Part print with two shaded views. Sizes in mm from the minimum x, y, z corner. A direction names the side the tool comes from. Give positions to 0.01 mm unless a question says otherwise; leave off trailing zeros. Order: outer loops, then holes, each group sorted by start corner. A loop starts at its lowest first (then second) coordinate and runs counter-clockwise, first axis right, second up. Notation, with made-up numbers: (-19.75, 84.25) -> (3.25, 84.25) arc R13 cw to (3.25, 108.25) -> close; hole circle Ø4 at (-10.75, 46). An arc over 180 degrees is marked (long way). Write item = value, one per line. Start each with the question number.
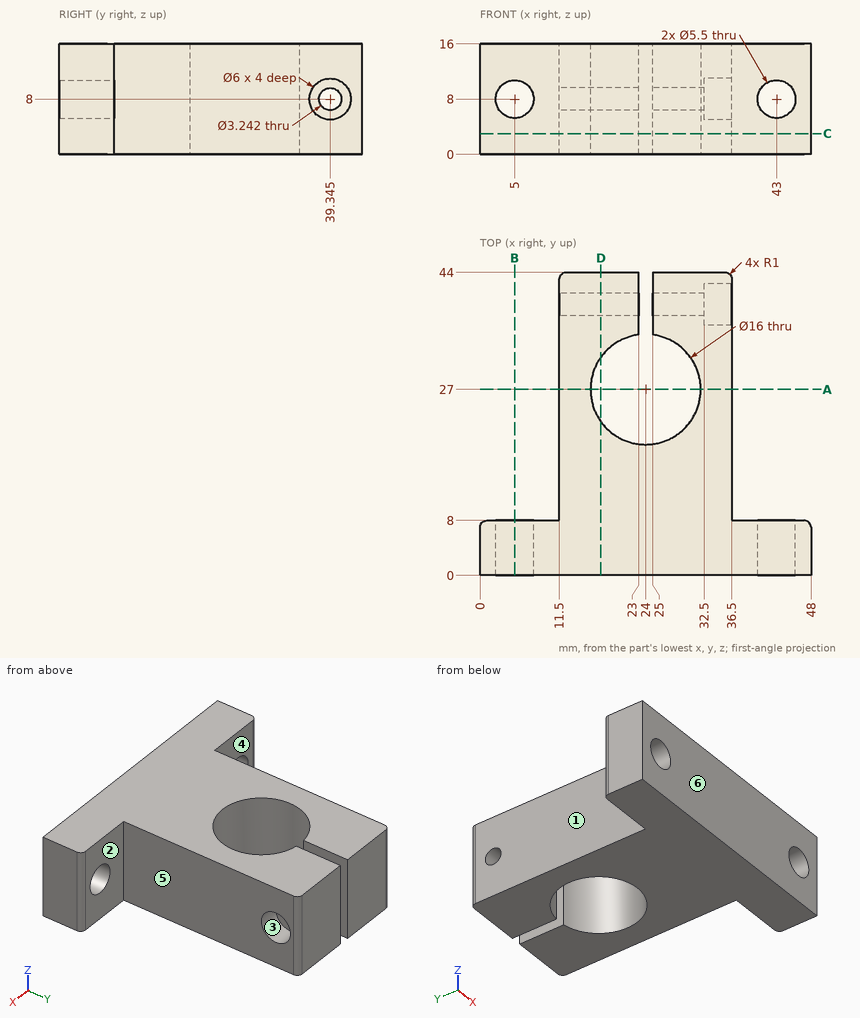
(1) Cut at C-C, the plane z = 3. Give the cut face in (x, y).
(2) Wall check: line 1 (X direction, y = 6, z = 8); line 2 (Y direction, x = 35.1, z = 8) (1 decimal); line 3 (Y direction, x = 25.5, z = 7.75). Give the ranges that are in metal, low to high. Write a range as [from, to].
(3) Mould opens along Y. For the marked faces 1, 2 and 3 say: released by +Y, released by -Y, zero draft, split by the parting line, or undercut.
(4) 3-axis set-ups, long thin cutter, end or side, ignore diameter. For the marked faces 4, 5 and 6: which of +Z, -Z, +X, -X, +Y, -Y reach the whole face in a straight line?
(5) Cut at B-B, the plane x = 5. Give the cut face in (y, z), plus the area to 3 significant figures.
(6) Cut at D-D, the plane x = 17.5. Give the cut face in (y, z) (1 decimal).
(7) Cut at A-A, the plane y = 27. Give the cut face in (x, z).
(8) Flat gauge pins, fed straight in: P1, Ø1.8, axis at y = 40, z = 8.5, coming from the +X side; P2, Ø5.5, axis at y = 39.35, z = 8, coming from the -X side; P3, Ø6.5, axis at x = 43, z = 8, coming from the +Y side; P4, Ø6, axis at y = 6.5, z = 7, coming from the -X side. Where does each tip first touch, or does it go through?
Results:
q1.outline = (0, 0) -> (48, 0) -> (48, 7) arc R1 ccw to (47, 8) -> (36.5, 8) -> (36.5, 43) arc R1 ccw to (35.5, 44) -> (25, 44) -> (25, 34.94) arc R8 cw (long way) to (23, 34.94) -> (23, 44) -> (12.5, 44) arc R1 ccw to (11.5, 43) -> (11.5, 8) -> (1, 8) arc R1 ccw to (0, 7) -> close
q2.line_1 = [0, 2.25], [7.75, 40.25], [45.75, 48]
q2.line_2 = [0, 36.3], [42.3, 44]
q2.line_3 = [0, 19.14], [34.86, 37.74], [40.95, 44]
q3.face_1 = zero draft
q3.face_2 = released by +Y
q3.face_3 = undercut
q4.face_4 = +Z, -Z, -X, +Y
q4.face_5 = +Z, -Z, +X, +Y
q4.face_6 = +Z, -Z, +X, -X, -Y
q5.outline = (0, 0) -> (8, 0) -> (8, 5.25) -> (0, 5.25) -> close; (0, 10.75) -> (8, 10.75) -> (8, 16) -> (0, 16) -> close
q5.area = 84.0 mm2
q6.outline = (0, 0) -> (22.3, 0) -> (22.3, 16) -> (0, 16) -> close; (31.7, 0) -> (44, 0) -> (44, 16) -> (31.7, 16) -> close; hole circle Ø3.2 at (39.3, 8)
q7.outline = (11.5, 0) -> (16, 0) -> (16, 16) -> (11.5, 16) -> close; (32, 0) -> (36.5, 0) -> (36.5, 16) -> (32, 16) -> close
q8.P1 = 32.5
q8.P2 = 11.5
q8.P3 = 8
q8.P4 = 0
